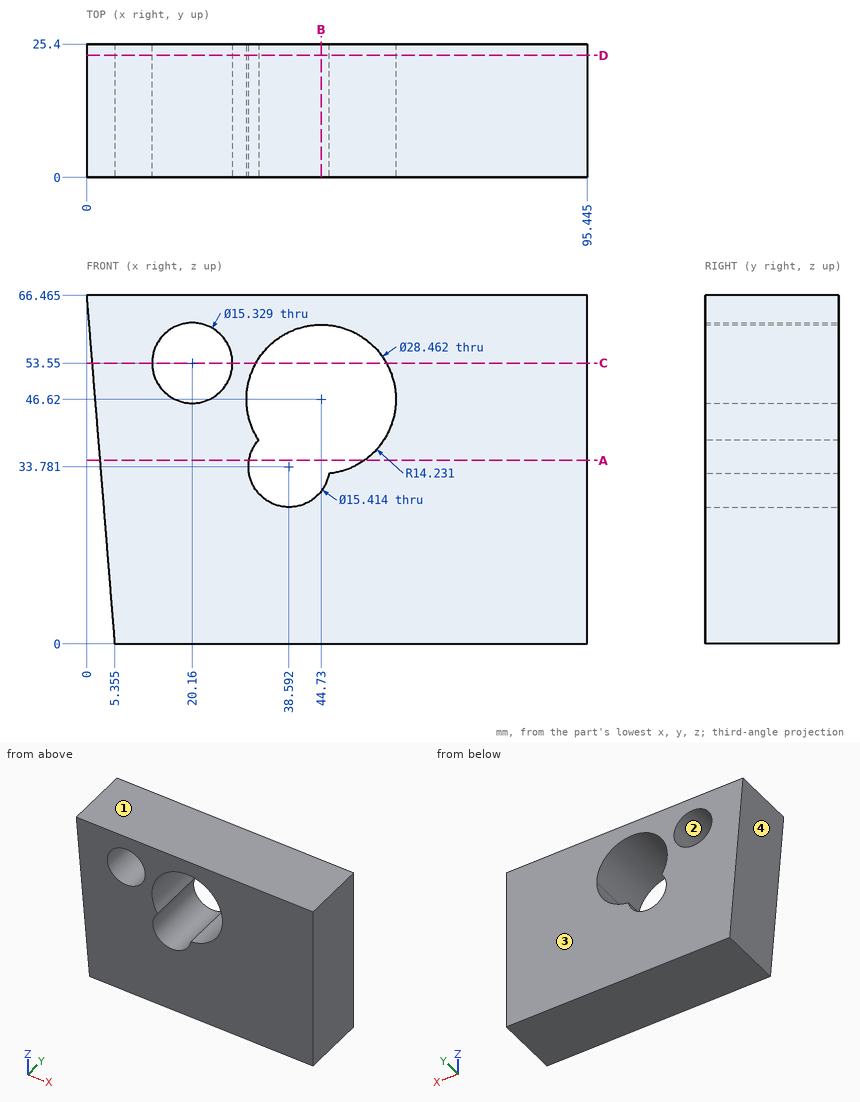
Drawing for the job (mm, zero at the part's lowest x, y, z). Round coordinates to 2 decimals unless told otherwise and drop trailing zeros. Order: outer loops, then holes, each group sorted by start corner. A loop starts at its lowest first (then second) coordinate and runs counter-clockwise, first axis right, second up. Notation, with made-up numbers: (-13.5, -22.5) -> (38.5, -22.5) arc R22 ccw to (38.5, -11.5) -> close; hole circle Ø8 at (45.5, 19.5). An arc over 180 degrees is marked (long way). Put each result on its own line as item: value.
Q1. Pull direction Z, two halves, no side cores. Call the marked faces 1, 2, 3 and 4: pulls with the +Z half, pulls with the -Z half, needs draft (parallel to the pull), parting line crosses it, or undercut.
From the geometry:
face 1: pulls with the +Z half
face 2: undercut
face 3: needs draft
face 4: pulls with the -Z half
Q2. Wall check: line 1 (X direction, y = 11, z = 48.5) (1 decimal); line 2 (X direction, y = 16.5, z = 58) (1 decimal); line 3 (X direction, y = 14, z = 36) (1 decimal). Give the ranges that are in metal, low to high. Write a range as [from, to].
From the geometry:
line 1: x = [1.4, 14.4], [25.9, 30.6], [58.8, 95.4]
line 2: x = [0.7, 13.9], [26.4, 36.2], [53.3, 95.4]
line 3: x = [2.5, 31.2], [54.2, 95.4]
Q3. Band-saw the part on A-A (z = 35). Give the cut face in (x, y) (1 decimal).
From the geometry:
outline: (2.5, 0) -> (31, 0) -> (31, 25.4) -> (2.5, 25.4) -> close; (52.9, 0) -> (95.4, 0) -> (95.4, 25.4) -> (52.9, 25.4) -> close
Q4. Band-saw the part on C-C (z = 53.55). Give the cut face in (x, y) (1 decimal).
From the geometry:
outline: (1, 0) -> (12.5, 0) -> (12.5, 25.4) -> (1, 25.4) -> close; (27.8, 0) -> (32.3, 0) -> (32.3, 25.4) -> (27.8, 25.4) -> close; (57.2, 0) -> (95.4, 0) -> (95.4, 25.4) -> (57.2, 25.4) -> close
Q5. Band-saw the part on B-B (x = 44.73). Give the cut face in (y, z) (1 decimal).
From the geometry:
outline: (0, 0) -> (25.4, 0) -> (25.4, 29.1) -> (0, 29.1) -> close; (0, 60.9) -> (25.4, 60.9) -> (25.4, 66.5) -> (0, 66.5) -> close
Q6. Pin check, flat tip, straight feed: pin 1 Ø17.5 at (x, z) = (20.16, 53.55) entering from +Y. Stop position of the tip, or through.
From the geometry:
pin 1: stops at y = 25.4
Q7. Band-saw the part on D-D (y = 23.25). State how many separate pieces and enclosed holes the cut face has, and give its area (3 significant figures).
From the geometry:
separate pieces: 1
enclosed holes: 2
area: 5,240 mm2
